The model under review builds one solid part; all positions refer to its coordinate system, in mm. A direction names the side the tool comes from. Round coordinates to 2 decimals unless told otherwise and drop trailing zeros. Write each loop counter-clockwise with the first axis right and the second up, starting at its lowest first coordinate (ties: lowest second). Pieces come first, ordered by that corner, then holes. Notation, with made-up numbers: (14, 67.5) -> (52, 67.5) arc R34 cw to (52, 99.5) -> close; hole circle Ø4 at (30, 5.5). An arc over 180 degrees is marked (long way). Answer as a JSON object with one key per item and string values. Group by question number.
1) Machinability: for faces 4 (the flat face through (129.5, 105, 98)), 5 (the flat face through (3, 51, 71)), 6 (the flat face through (149, 83, 94)), 7 (the flat face through (1, 37, 83.5)), which of the approach directions +Z, -Z, +X, -X, +Y, -Y give a long, thin tool a straight path to every point of the face, cutting with its end or side? Answer none if there is none.
2) Mouldability with a two-part tool opening along Z and no side actions: class faces 1 (the cylindrical face through (75, 106, 101)), 2 (the flat face through (76, 97, 71)), 3 (the flat face through (74, 51, 43)) as pulls with the +Z half, pulls with the -Z half, needs draft (parallel to the pull), parting line crosses it, or undercut.
3) We need section C-C, the plane x = 54. Write out the cut boundary in (y, z).
4) We need section A-A, the plane z = 63. Write out the cut boundary in (x, y).
5) Insertion check: pin 1 Ø14.5 at (x, y) = (16, 15) entering from +Z; pin 2 Ø4 at (x, z) = (108, 55) entering from -Y; pin 3 Ø2.5 at (y, z) = (104, 96.5) entering from -X; pin 4 Ø2.5 at (y, z) = (103, 96) entering from +X. Each pin has a flat end and moves straight along its axis. Give the tip position at first contact, or say it passes through.
6) We need section B-B, the plane y = 38. Write out the cut boundary in (x, z).
7) We need section D-D, the plane z = 92.5. Count the separate pieces of the cut face and the enclosed holes in it, then the cut area to 3 significant figures.
8) To check wall thickness, follow probe 1 along X at (y, z) = (32.5, 81.5); probe 2 along Y at (x, z) = (100.5, 49); probe 3 along Z at (x, y) = (95.5, 12). State the ranges of each line that lie inside material, in increasing order. Write a range as [from, to].
Autodesk Fusion 360 part; units mm, degrees
sketch "草图1" plane through (75, 0, 0) normal (1, 0, 0) x (0, 1, 0)
  line L0 (100, 100) -> (103, 100)
  line L1 (103, 100) -> (103, 103.5)
  line L2 (105.5, 106) -> (106.5, 106)
  line L3 (109, 103.5) -> (109, 100)
  line L4 (108.7423, 99.3777) -> (100, 90.6355)
  circle A0 centre (106, 103) radius 2
  line L5 (100, 0) -> (100, 100)
  arc A1 (105.5, 106) -> (103, 103.5) centre (105.5, 103.5) ccw
  arc A2 (109, 103.5) -> (106.5, 106) centre (106.5, 103.5) ccw
  arc A3 (108.7423, 99.3777) -> (109, 100) centre (108.12, 100) ccw
  point P0 (100, 100)
  dimension "d1" = 3
  dimension "d2" = 4
  dimension "d3" = 3
  dimension "d6" = 3
  dimension "d9" = 3
  dimension "d10" = 3
  dimension "d13" = 135
  dimension "d14" = 2.5
  dimension "d15" = 2.5
  dimension "d16" = 0.88
sketch "草图2" plane through (18, 0, 0) normal (1, 0, 0) x (0, 1, 0)
  arc A0 (108.7423, 99.3777) -> (109, 100) centre (108.12, 100) ccw
  arc A1 (105.5, 106) -> (103, 103.5) centre (105.5, 103.5) ccw
  line L0 (105.5, 106) -> (106.5, 106)
  line L1 (100, 100) -> (103, 100)
  arc A2 (109, 103.5) -> (106.5, 106) centre (106.5, 103.5) ccw
  circle A3 centre (106, 103) radius 2
  line L2 (109, 103.5) -> (109, 100)
  line L3 (108.7423, 99.3777) -> (100, 90.6355)
  line L4 (103, 100) -> (103, 103.5)
  line L5 (100, 0) -> (100, 100)
  point P0 (100, 100)
  point P1 (100, 100)
  point P2 (100, 100)
  dimension "d17" = 3
  dimension "d18" = 4
  dimension "d21" = 3
  dimension "d22" = 3
  dimension "d23" = 3
  dimension "d26" = 3
  dimension "d27" = 135
  dimension "d30" = 2.5
  dimension "d31" = 2.5
  dimension "d32" = 0.88
sketch "草图3" plane through (147, 0, 0) normal (-1, 0, 0) x (0, -1, 0)
  line L0 (-59, 100) -> (-59, 87)
  line L1 (-59, 87) -> (-83, 87)
  line L2 (-83, 87) -> (-83, 100)
  line L3 (-83, 100) -> (-97, 100)
  line L4 (-97, 100) -> (-97, 3)
  line L5 (-97, 3) -> (-3, 3)
  line L6 (-3, 3) -> (-3, 100)
  line L7 (-3, 100) -> (-59, 100)
  line L8 (-8, 100) -> (-3, 100)
  line L9 (-3, 100) -> (-3, 90)
  line L10 (-3, 90) -> (-8, 90)
  line L11 (-8, 90) -> (-8, 100)
  dimension "d33" = 5
  dimension "d34" = 10
sketch "草图4" plane through (132, 0, 0) normal (-1, 0, 0) x (0, -1, 0)
  line L0 (-100, 100) -> (-103, 100)
  line L1 (-105.5, 106) -> (-106.5, 106)
  arc A0 (-106.5, 106) -> (-109, 103.5) centre (-106.5, 103.5) ccw
  line L2 (-103, 100) -> (-103, 103.5)
  arc A1 (-103, 103.5) -> (-105.5, 106) centre (-105.5, 103.5) ccw
  circle A2 centre (-106, 103) radius 2
  line L3 (-109, 103.5) -> (-109, 100)
  arc A3 (-109, 100) -> (-108.7657, 99.4343) centre (-108.2, 100) ccw
  line L4 (-108.7657, 99.4343) -> (-100, 90.6686)
  line L5 (-100, 0) -> (-100, 100)
  point P0 (-105.9337, 94.2405)
  point P1 (-105.9337, 94.2405)
  point P2 (-100, 100)
  dimension "d35" = 3.5
  dimension "d36" = 3
  dimension "d37" = 3
  dimension "d38" = 3
  dimension "d39" = 3
  dimension "d42" = 3
  dimension "d43" = 1
  dimension "d44" = 4
  dimension "d45" = 0.8
  dimension "d46" = 135
sketch "草图5" plane through (0, 0, 0) normal (0, -1, 0) x (1, 0, 0)
  line L0 (0, 0) -> (150, 0)
  line L1 (150, 0) -> (150, 100)
  line L2 (150, 100) -> (0, 100)
  line L3 (0, 100) -> (0, 0)
  line L4 (63, 100) -> (87, 100)
  line L5 (87, 100) -> (87, 76)
  line L6 (87, 76) -> (63, 76)
  line L7 (63, 76) -> (63, 100)
  dimension "d47" = 24
  dimension "d48" = 24
sketch "草图6" plane through (0, 0, 0) normal (-1, 0, 0) x (0, -1, 0)
  line L0 (-100, 0) -> (0, 0)
  line L1 (0, 0) -> (0, 100)
  line L2 (0, 100) -> (-100, 100)
  line L3 (-100, 100) -> (-100, 0)
  line L4 (-71, 100) -> (-54.5, 100)
  line L5 (-54.5, 100) -> (-54.5, 83.5)
  line L6 (-54.5, 83.5) -> (-71, 83.5)
  line L7 (-71, 83.5) -> (-71, 100)
  line L8 (-45.5, 100) -> (-29, 100)
  line L9 (-29, 100) -> (-29, 83.5)
  line L10 (-29, 83.5) -> (-45.5, 83.5)
  line L11 (-45.5, 83.5) -> (-45.5, 100)
  line L12 (-54.5, 100) -> (-45.5, 100) construction
  line L13 (-54.5, 100) -> (-45.5, 100)
  line L14 (-45.5, 100) -> (-45.5, 97.5)
  line L15 (-45.5, 97.5) -> (-54.5, 97.5)
  line L16 (-54.5, 97.5) -> (-54.5, 100)
  dimension "d49" = 16.5
  dimension "d50" = 16.5
  dimension "d51" = 16.5
  dimension "d52" = 16.5
  dimension "d53" = 9
  dimension "d56" = 14
sketch "草图7" plane through (0, 0, 3) normal (0, 0, 1) x (-1, 0, 0)
  line L0 (0, -100) -> (0, 0)
  line L1 (0, 0) -> (-150, 0)
  line L2 (-150, 0) -> (-150, -100)
  line L3 (-150, -100) -> (0, -100)
  line L4 (-3, -3) -> (-147, -3)
  line L5 (-147, -3) -> (-147, -97)
  line L6 (-147, -97) -> (-3, -97)
  line L7 (-3, -97) -> (-3, -3)
  dimension "d57" = -3
sketch "草图8" plane through (150, 0, 0) normal (1, 0, 0) x (0, 1, 0)
  line L0 (0, 0) -> (100, 0)
  line L1 (100, 0) -> (100, 100)
  line L2 (100, 100) -> (0, 100)
  line L3 (0, 100) -> (0, 0)
  line L4 (59, 100) -> (83, 100)
  line L5 (83, 100) -> (83, 87)
  line L6 (83, 87) -> (59, 87)
  line L7 (59, 87) -> (59, 100)
  dimension "d58" = 24
  dimension "d59" = 13
  dimension "d60" = 17
sketch "草图9" plane through (0, 0, 0) normal (0, 0, 1) x (1, 0, 0)
  line L0 (0, 0) -> (150, 0)
  line L1 (150, 0) -> (150, 100)
  line L2 (150, 100) -> (0, 100)
  line L3 (0, 100) -> (0, 0)
  dimension "d61" = 150
  dimension "d62" = 100
extrude "拉伸1" add sketch "草图9" along normal blind 3
extrude "拉伸2" add sketch "草图7" along normal blind 97
extrude "拉伸3" cut sketch "草图5" against normal blind 25 contours L2 L4 L5 L6 L7
extrude "拉伸4" cut sketch "草图6" against normal blind 10 contours L2 L4 L5 L6 L7 L16 | L2 L8 L9 L10 L11 L14 | L2 L5 L11 L13 L14 L15 L16
extrude "拉伸5" cut sketch "草图8" against normal blind 20 contours L2 L4 L5 L6 L7
extrude "拉伸6" cut sketch "草图3" against normal blind 10 contours L6 L7 L8 L9 L10 L11
extrude "拉伸7" add sketch "草图1" along normal mid plane 5
extrude "拉伸8" add sketch "草图2" along normal mid plane 5
extrude "拉伸9" add sketch "草图4" along normal mid plane 5
extrude "拉伸10" add 1 faces at (51, 65.6667, 3) along direction (0, 0, 1) blind 40
extrude "拉伸11" cut 1 faces at (50, 66.6667, 0) along direction (0, 0, 1) blind 40
equation "d7 = 100 mm - 3 mm"
Here are the results:
{
 "1": {"face 4": "+Z, -Z, +Y", "face 5": "+Z", "face 6": "+Z, +X", "face 7": "+Z, -X"},
 "2": {"face 1": "undercut", "face 2": "needs draft", "face 3": "pulls with the +Z half"},
 "3": {"outline": "(0, 40) -> (100, 40) -> (100, 100) -> (97, 100) -> (97, 43) -> (3, 43) -> (3, 100) -> (0, 100) -> close"},
 "4": {"outline": "(0, 0) -> (150, 0) -> (150, 100) -> (0, 100) -> close; hole (3, 3) -> (147, 3) -> (147, 97) -> (3, 97) -> close"},
 "5": {"pin 1": "stops at z = 43", "pin 2": "stops at y = 0", "pin 3": "stops at x = 15.5", "pin 4": "stops at x = 134.5"},
 "6": {"outline": "(0, 40) -> (150, 40) -> (150, 100) -> (147, 100) -> (147, 43) -> (3, 43) -> (3, 83.5) -> (0, 83.5) -> close"},
 "7": {"separate pieces": "5", "enclosed holes": "0", "area": "1,230 mm^2"},
 "8": {"probe 1": "x = [0, 3], [147, 150]", "probe 2": "y = [0, 3], [97, 100]", "probe 3": "z = [40, 43]"}
}
